Geometry check sheet. Reference: the model listing, model coordinates, mm. A direction names the side the tool comes from. Coordinates: 2 decimals unless noted, no trailing zeros. Order: outer loops, then holes, each group sorted by start corner. A loop starts at its lowest first (then second) coordinate and runs counter-clockwise, first axis right, second up. Notation, with made-up numbers: (-31.75, 23) -> (1.25, 23) arc R27 ccw to (1.25, 54) -> close; hole circle Ø5 at (14, 61.25). An arc over 180 degrees is marked (long way). Answer as CSV lines item,"result". Start each with the question number.
from build123d import *

# Parameters (mm, degrees)
F0_W      = 120
F0_H      = 29
F1_DEPTH  = 5
F2_W      = 120
F2_H      = 10
F3_DEPTH  = 2.5
F5_DEPTH  = 2
F6_R      = 1.5
F7_DEPTH  = 25
F8_W      = 15.2
F8_H      = 1.875
F8_W_2    = 12.8
F9_DEPTH  = 18
F10_W     = 7.5
F10_H     = 1
F11_DEPTH = 3.001


with BuildPart() as f1:
    # F0 (on Top) → F1 (new body)
    with BuildSketch(Plane.XY):
        with Locations((-5.830355, 0.973214)):
            Rectangle(F0_W, F0_H)
    extrude(amount=F1_DEPTH)

    # F2 (on face) → F3 (cut)
    with BuildSketch(Plane.XY.offset(5)):
        with Locations((-5.830355, 7.473214)):
            Rectangle(F2_W, F2_H)
        with Locations((-5.830355, -5.526786)):
            Rectangle(F2_W, F2_H)
    extrude(amount=-F3_DEPTH, mode=Mode.SUBTRACT)

    # F4 (on face) → F5 (join)
    with BuildSketch(Plane(origin=(0, 15.473214, 0), x_dir=(-1, 0, 0), z_dir=(0, 1, 0))):
        Polygon((45.830355, 5), (65.830355, 5), (65.830355, 29), (45.830355, 29), (45.830355, 19), (27.830355, 19), (27.830355, 5), align=None)
    extrude(amount=-F5_DEPTH)

    # F6 (on face) → F7 (cut)
    with BuildSketch(Plane(origin=(0, 15.473214, 0), x_dir=(-1, 0, 0), z_dir=(0, 1, 0))):
        with Locations((57.830355, 21.5)):
            Circle(F6_R)
        with Locations((34.830355, 9)):
            Circle(F6_R)
    extrude(amount=-F7_DEPTH, mode=Mode.SUBTRACT)

    # F8 (on face) → F9 (cut)
    with BuildSketch(Plane(origin=(0, 15.473214, 0), x_dir=(-1, 0, 0), z_dir=(0, 1, 0))):
        with Locations((39.430355, 4.0625)):
            Rectangle(F8_W, F8_H)
        with Locations((56.430355, 4.0625)):
            Rectangle(F8_W_2, F8_H)
    extrude(amount=-F9_DEPTH, mode=Mode.SUBTRACT)

    # F10 (on face) → F11 (cut, through all)
    with BuildSketch(Plane(origin=(0, -10.526786, 0), x_dir=(-1, 0, 0), z_dir=(0, 1, 0))):
        with Locations((39.330355, 3.625)):
            Rectangle(F10_W, F10_H)
    extrude(amount=-F11_DEPTH, mode=Mode.SUBTRACT)


solid = f1.part
Q1. Release check for a two-part mould opening along Y. For faces 1 (the flat face through (7, -0.527, 4)), 2 (the flat face through (-56, 1, 3.125)), 3 (the flat face through (-7, -13.527, 2)) record: released by +Y, released by -Y, zero draft, split by the parting line, or undercut.
Q2. Sectioned sample at D-D, the plane x = 7. Record the cut outline in (y, z), then the cut area to 3 significant figures.
Q3. Sectioned sample at A-A, the plane z = 21.5. Record the cut outline in (x, y).
Q4. Access from +Z, -Z, +X, -X, +Y, -Y to the whole of each face (thin tool, end or side, straight path). Record for faces 4 (the flat face through (-49, 1, 5)), 5 (the flat face through (-7, -10.527, 4)), 6 (the flat face through (-39, -12, 4.125)), 7 (the flat face through (-39, 14, 5)).
Q5. Go/stop test with flat-tipped pins: pin 1 Ø7 at (x, z) = (-44.5, 19) entering from -Y; pin 2 Ø1.5 at (x, y) = (-63.5, 1.5) entering from +Z; pin 3 Ø1.5 at (x, y) = (-58, 0.5) entering from +Z (3 decimals); pin 4 Ø10 at (x, y) = (25.5, 5) entering from -Z. Record where each tip stops, or that it passes through.
Q6. Sectioned sample at B-B, the plane x = -57.5. Record the cut outline in (y, z) (3 decimals), then the cut area to 3 significant figures.
Q7. Thickness scan on L1, parallel to Y at x = 28, z = 3.5; L2, parallel to Z at x = -1, y = 9.5; L3, parallel to X at y = 14.25, z = 7. Record the ranges inside material, lowest first.
Q8. Sectioned sample at C-C, the plane y = 0.5. Record the cut outline in (x, z) (3 decimals).
Geometry results:
1,face 1,"undercut"
1,face 2,"zero draft"
1,face 3,"released by -Y"
2,outline,"(-13.53, 0) -> (15.47, 0) -> (15.47, 5) -> (12.47, 5) -> (12.47, 2.5) -> (2.47, 2.5) -> (2.47, 5) -> (-0.53, 5) -> (-0.53, 2.5) -> (-10.53, 2.5) -> (-10.53, 5) -> (-13.53, 5) -> close"
2,area,"95.0 mm^2"
3,outline,"(-65.83, 13.47) -> (-59.33, 13.47) -> (-59.33, 15.47) -> (-65.83, 15.47) -> close; (-56.33, 13.47) -> (-45.83, 13.47) -> (-45.83, 15.47) -> (-56.33, 15.47) -> close"
4,face 4,"+Z, +X, -X, -Y"
4,face 5,"+Z, +X, -X"
4,face 6,"+Y, -Y"
4,face 7,"+Y"
5,pin 1,"stops at y = 13.47"
5,pin 2,"stops at z = 5"
5,pin 3,"stops at z = 3.125"
5,pin 4,"stops at z = 0"
6,outline,"(-13.527, 0) -> (15.473, 0) -> (15.473, 3.125) -> (12.473, 3.125) -> (12.473, 2.5) -> (2.473, 2.5) -> (2.473, 3.125) -> (-0.527, 3.125) -> (-0.527, 2.5) -> (-10.527, 2.5) -> (-10.527, 5) -> (-13.527, 5) -> close; (13.473, 5) -> (15.473, 5) -> (15.473, 20.037) -> (13.473, 20.037) -> close; (13.473, 22.963) -> (15.473, 22.963) -> (15.473, 29) -> (13.473, 29) -> close"
6,area,"126 mm^2"
7,L1,"y = -13.53 to -10.53, -0.53 to 2.47, 12.47 to 15.47"
7,L2,"z = 0 to 2.5"
7,L3,"x = -65.83 to -27.83"
8,outline,"(-65.83, 0) -> (54.17, 0) -> (54.17, 5) -> (-31.83, 5) -> (-31.83, 3.125) -> (-47.03, 3.125) -> (-47.03, 5) -> (-50.03, 5) -> (-50.03, 3.125) -> (-62.83, 3.125) -> (-62.83, 5) -> (-65.83, 5) -> close"
